Verification items for this drawing (mm, ordinates from the low corner). Coordinates: 2 decimals unless noted, no trailing zeros. Order: outer loops, then holes, each group sorted by start corner. A loop starts at its lowest first (then second) coordinate and runs counter-clockwise, first axis right, second up. Notation, with made-up numbers: M -27.75,5 L -2.75,5 A26 cw -2.75,43 Z; hole C -3,32 d7. An arc over 180 degrees is marked long. Return JSON: item names as keys, results as strings. Group by question number.
1. Section check C-C, the plane y = 0.7. Record the cut outline in (x, z) (3 decimals).
2. Section check A-A, the plane x = 56. Record the cut outline in (y, z).
3. Section check D-D, the plane x = 30. Record the cut outline in (y, z) (3 decimals), plus the area to 4 significant figures.
4. Section check B-B, the plane z = 4. Record the cut outline in (x, y), plus the area to 3 significant figures.
5. Material ranges on line 1 along Z through (x, y) = (56, 0.25); line 2 along X through (y, z) = (0.7, 56); line 3 along Z through (x, y) = (30, 0.3) (3 decimals), recorded low to high.
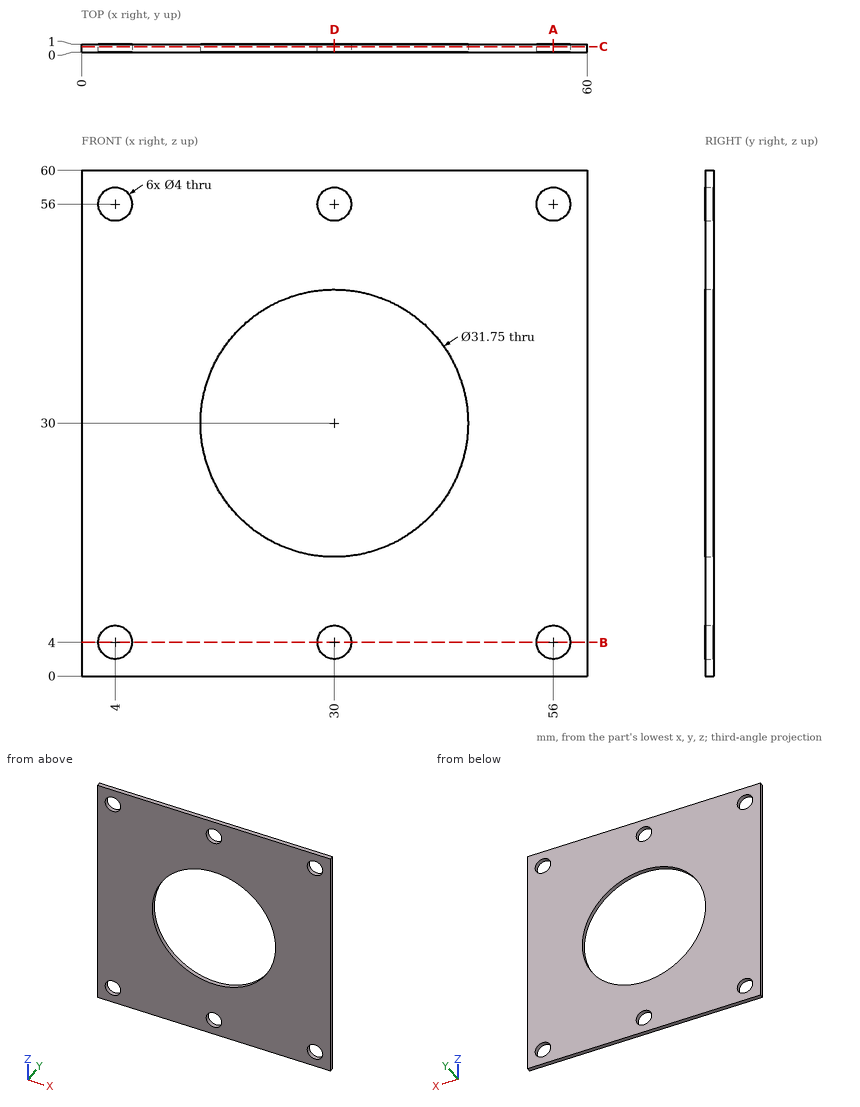
Answers follow:
{
 "1": {"outline": "M 0,0 L 60,0 L 60,60 L 0,60 Z; hole C 4,4 d4; hole C 4,56 d4; hole C 30,30 d31.75; hole C 30,4 d4; hole C 30,56 d4; hole C 56,4 d4; hole C 56,56 d4"},
 "2": {"outline": "M 0,0 L 1,0 L 1,2 L 0,2 Z; M 0,6 L 1,6 L 1,54 L 0,54 Z; M 0,58 L 1,58 L 1,60 L 0,60 Z"},
 "3": {"outline": "M 0,0 L 1,0 L 1,2 L 0,2 Z; M 0,6 L 1,6 L 1,14.125 L 0,14.125 Z; M 0,45.875 L 1,45.875 L 1,54 L 0,54 Z; M 0,58 L 1,58 L 1,60 L 0,60 Z", "area": "20.25 mm^2"},
 "4": {"outline": "M 0,0 L 2,0 L 2,1 L 0,1 Z; M 6,0 L 28,0 L 28,1 L 6,1 Z; M 32,0 L 54,0 L 54,1 L 32,1 Z; M 58,0 L 60,0 L 60,1 L 58,1 Z", "area": "48.0 mm^2"},
 "5": {"line 1": "0 to 2, 6 to 54, 58 to 60", "line 2": "0 to 2, 6 to 28, 32 to 54, 58 to 60", "line 3": "0 to 2, 6 to 14.125, 45.875 to 54, 58 to 60"}
}
